Source: CAD feature listing. Evaluate the final solid. Frame: model axes, mm. Give positions to 0.01 mm unless a question says otherwise; leave off trailing zeros. Order: outer loops, then holes, each group sorted by start corner. A loop starts at its lowest first (then second) coordinate and runs counter-clockwise, first axis right, second up. Notation, with made-up numbers: (-31.75, 64.5) - (-0.75, 64.5) arc R15 cw to (-0.75, 82.5) - close; hole circle Ø4 at (37, 52.25). An arc over 180 degrees is marked (long way). Use CSV: the item, a comma, the result in double quotes.
```python
from build123d import *

# Parameters (mm, degrees)
F0_R     = 1.4732
F1_DEPTH = 3.175


# Not quite as in the source:
# - a length typed as a fraction of an inch, garbled in the dataset ("3 / 203.2 mm" for 3/8 in), is restored


with BuildPart() as f1:
    # F0 (on Top) → F1 (new body)
    with BuildSketch(Plane.XY):
        with BuildLine():
            Line((6.35, -19.05), (6.35, 25.4))
            Line((6.35, 25.4), (6.35, 31.75))
            ThreePointArc((6.35, 31.75), (4.4901280605, 36.2401280605), (0, 38.1))
            ThreePointArc((0, 38.1), (-4.4901280605, 36.2401280605), (-6.35, 31.75))
            Line((-6.35, 31.75), (-6.35, 25.4))
            Line((-6.35, 25.4), (-6.35, -19.05))
            ThreePointArc((-6.35, -19.05), (-4.4901280605, -23.5401280605), (0, -25.4))
            ThreePointArc((0, -25.4), (4.4901280605, -23.5401280605), (6.35, -19.05))
        make_face()
        with Locations((0, -19.05)):
            Circle(F0_R, mode=Mode.SUBTRACT)
        with Locations((0, 19.05)):
            Circle(F0_R, mode=Mode.SUBTRACT)
    extrude(amount=F1_DEPTH)


solid = f1.part
```
Item 1: Mould query, pull axis Y, two halves, no side actions, for faces 1 (the cylindrical face through (-0.19, -17.59, 1.57)), 2 (the flat face through (0, 7, 0)). Classes: released by +Y, released by -Y, zero draft, split by the parting line, or undercut.
Filled in:
face 1,"undercut"
face 2,"zero draft"
Item 2: Material intervals for line 1 (Y direction, x = 1, z = 2.3); line 2 (Y direction, x = -2.25, z = 0.4); line 3 (Y direction, x = 2.75, z = 3.05), sorted ascending. Write a range as from..to.
Filled in:
line 1,"y = -25.32..-20.13, -17.97..17.97, 20.13..38.02"
line 2,"y = -24.99..37.69"
line 3,"y = -24.77..37.47"
Item 3: Section C-C on x = 2.5. Return the cut outline in (y, z) (3 decimals).
Filled in:
outline,"(-24.887, 0) - (37.587, 0) - (37.587, 3.175) - (-24.887, 3.175) - close"
Item 4: Section A-A on y = 19.05. Return the cut outline in (x, z) (3 decimals), then the cut area to 3 significant figures.
Filled in:
outline,"(-6.35, 0) - (-1.473, 0) - (-1.473, 3.175) - (-6.35, 3.175) - close; (1.473, 0) - (6.35, 0) - (6.35, 3.175) - (1.473, 3.175) - close"
area,"31.0 mm2"
Item 5: First-contact query: pin 1 (1 mm diameter, centred on x = 2.5, z = 1.5, fed in from -Y). Flat tip, straight axial feed; report the tip coordinate or a pass-through.
Filled in:
pin 1,"stops at y = -25.08"
Item 6: Section D-D on x = 5. Return the cut outline in (y, z) (3 decimals), then the cut area to 3 significant figures.
Filled in:
outline,"(-22.964, 0) - (35.664, 0) - (35.664, 3.175) - (-22.964, 3.175) - close"
area,"186 mm2"
Item 7: Section B-B on z = 1.25. Return the cut outline in (x, y).
Filled in:
outline,"(-6.35, -19.05) arc R6.35 ccw to (6.35, -19.05) - (6.35, 31.75) arc R6.35 ccw to (-6.35, 31.75) - close; hole circle Ø2.95 at (0, -19.05); hole circle Ø2.95 at (0, 19.05)"
